Can you work these out from the model? Positions are in its coordinate system, mm. Round coordinates to 2 decimals unless told otherwise and drop trailing zeros. Write each loop counter-clockwise with the first axis right and the second up, starting at its lowest first coordinate (ties: lowest second). Pieces come first, ordered by that corner, then holes. Notation, with made-up numbers: M -38.5,3.25 L -31.5,3.25 A15 ccw -31.5,15.25 Z; hole C 0,80.5 d10. An arc over 180 degrees is marked long. Answer as a JSON object with one key per item and string values. Group by question number.
1) Suppose I cut it at A-A, the plane x = -11.5. Write out the boundary of the cut face in (y, z), and give its area (3 significant figures).
2) Suppose I cut it at C-C, the plane x = 14. Write out the boundary of the cut face in (y, z).
3) Please list where these lines run through material, in increasing order: L1, parallel to Z at x = 29.5, y = 4.75; L2, parallel to X at y = 2.5, z = -9.5 (3 decimals); L3, parallel to Z at x = -9, y = 5.5. Write a range as [from, to].
4) Suppose I cut it at D-D, the plane z = -8. Write out the boundary of the cut face in (x, y) (1 decimal).
5) I'm going to push a flat-ended pin straight in: pin 1 Ø2.5 at (x, z) = (44.32, -16.07) entering from -Y. Where does the tip first touch, or does it pass through?
6) Suppose I cut it at B-B, the plane z = -27. Write out the boundary of the cut face in (x, y) (1 decimal), and give its area (3 significant figures).
from build123d import *

# Parameters (mm, degrees)
SKETCH1_W           = 82.55
SKETCH1_H           = 43.18
SKETCH1_R           = 2.159
SKETCH1_W_2         = 40.64
SKETCH1_H_2         = 20.193
SKETCH1_W_3         = 25.4
SKETCH1_H_3         = 3.175
SKETCH1_W_4         = 6.0325
SKETCH1_H_4         = 19.05
BOSS_EXTRUDE1_DEPTH = 6.0325
SKETCH2_W           = 3.175
SKETCH2_H           = 6.35
CUT_EXTRUDE1_DEPTH  = 6.0325


with BuildPart() as part:
    # Sketch1 → Boss-Extrude1 (new body)
    with BuildSketch(Plane(origin=(0, 0, 0), x_dir=(1, 0, 0), z_dir=(0, 1, 0))):
        with Locations((20.32, 10.0965)):
            Rectangle(SKETCH1_W, SKETCH1_H)
        with Locations((44.323, 16.0655)):
            Circle(SKETCH1_R, mode=Mode.SUBTRACT)
        with Locations((44.323, 4.1275)):
            Circle(SKETCH1_R, mode=Mode.SUBTRACT)
        with Locations((-3.683, 4.1275)):
            Circle(SKETCH1_R, mode=Mode.SUBTRACT)
        with Locations((-3.683, 16.0655)):
            Circle(SKETCH1_R, mode=Mode.SUBTRACT)
        with Locations((20.32, 10.0965)):
            Rectangle(SKETCH1_W_2, SKETCH1_H_2, mode=Mode.SUBTRACT)
        with Locations((20.32, -6.35)):
            Rectangle(SKETCH1_W_3, SKETCH1_H_3, mode=Mode.SUBTRACT)
        with Locations((20.32, 26.543)):
            Rectangle(SKETCH1_W_3, SKETCH1_H_3, mode=Mode.SUBTRACT)
        with Locations((-11.6205, 10.0965)):
            Rectangle(SKETCH1_W_4, SKETCH1_H_4, mode=Mode.SUBTRACT)
        with Locations((52.2605, 10.0965)):
            Rectangle(SKETCH1_W_4, SKETCH1_H_4, mode=Mode.SUBTRACT)
    extrude(amount=BOSS_EXTRUDE1_DEPTH)

    # Sketch2 → Cut-Extrude1 (cut)
    with BuildSketch(Plane(origin=(0, 6.0325, 0), x_dir=(1, 0, 0), z_dir=(0, 1, 0))):
        with Locations((42.2275, 10.0965)):
            Rectangle(SKETCH2_W, SKETCH2_H)
    extrude(amount=-CUT_EXTRUDE1_DEPTH, mode=Mode.SUBTRACT)


solid = part.part
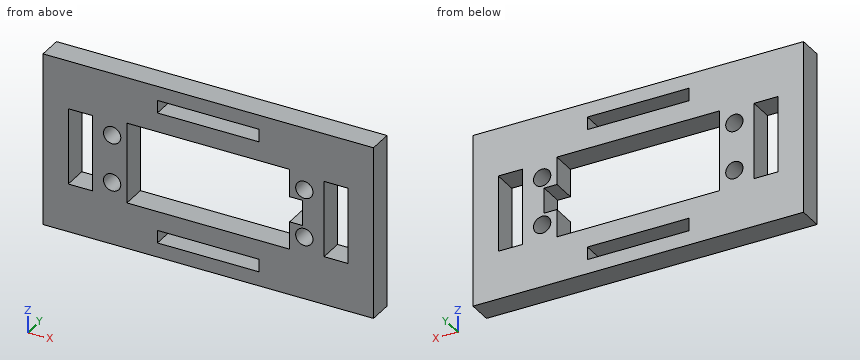
Results:
{
 "1": {"outline": "M 0,-31.69 L 6.03,-31.69 L 6.03,-19.62 L 0,-19.62 Z; M 0,-0.57 L 6.03,-0.57 L 6.03,11.49 L 0,11.49 Z", "area": "146 mm^2"},
 "2": {"outline": "M 0,-31.69 L 6.03,-31.69 L 6.03,-28.13 L 0,-28.13 Z; M 0,-24.96 L 6.03,-24.96 L 6.03,-20.19 L 0,-20.19 Z; M 0,0 L 6.03,0 L 6.03,4.76 L 0,4.76 Z; M 0,7.94 L 6.03,7.94 L 6.03,11.49 L 0,11.49 Z"},
 "3": {"L1": "[-31.69, -28.13], [-24.96, -20.19], [0, 4.76], [7.94, 11.49]", "L2": "[-20.955, -14.637], [-8.604, 0], [43.815, 49.244], [55.277, 61.595]", "L3": "[-31.69, -19.62], [-0.57, 11.49]"},
 "4": {"outline": "M -21,0 L -14.6,0 L -14.6,6 L -21,6 Z; M -8.6,0 L 0,0 L 0,6 L -8.6,6 Z; M 43.8,0 L 49.2,0 L 49.2,6 L 43.8,6 Z; M 55.3,0 L 61.6,0 L 61.6,6 L 55.3,6 Z"},
 "5": {"pin 1": "through"},
 "6": {"outline": "M -21,0 L 7.6,0 L 7.6,6 L -21,6 Z; M 33,0 L 61.6,0 L 61.6,6 L 33,6 Z", "area": "345 mm^2"}
}
